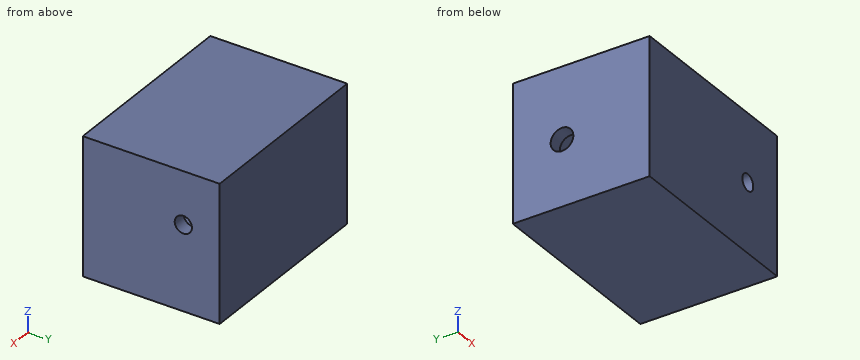
```python
from build123d import *

# Parameters (mm, degrees)
SKETCH1_W           = 70
SKETCH1_H           = 50
BOSS_EXTRUDE1_DEPTH = 50
CUT_EXTRUDE1_START  = -5
SKETCH2_W           = 60
SKETCH2_H           = 40
CUT_EXTRUDE1_DEPTH  = 40
CUT_EXTRUDE2_REACH  = 81.52
SKETCH3_R           = 3
CUT_EXTRUDE3_REACH  = 92.673
SKETCH4_R           = 3.149743794
CUT_EXTRUDE4_REACH  = 92.673
SKETCH5_R           = 4.144549467


with BuildPart() as part:
    # Sketch1 → Boss-Extrude1 (new body)
    with BuildSketch(Plane.XY):
        with Locations((-7.408376963, -3.664921466)):
            Rectangle(SKETCH1_W, SKETCH1_H)
    extrude(amount=BOSS_EXTRUDE1_DEPTH)

    # Sketch2 → Cut-Extrude1 (cut)
    with BuildSketch(Plane(origin=(0, 0, 0), x_dir=(-1, 0, 0), z_dir=(0, 0, -1)).offset(CUT_EXTRUDE1_START)):
        with Locations((7.408376963, -3.664921466)):
            Rectangle(SKETCH2_W, SKETCH2_H)
    extrude(amount=-CUT_EXTRUDE1_DEPTH, mode=Mode.SUBTRACT)

    # Sketch3 → Cut-Extrude2 (cut, up to next)
    with BuildSketch(Plane(origin=(0, -23.664921466, 0), x_dir=(1, 0, 0), z_dir=(0, 1, 0)), mode=Mode.PRIVATE) as cut_extrude2_sk1:
        with Locations(Location((11.436283644, -25.254491461, 0), (0, 0, 270))):
            Circle(SKETCH3_R)
    cut_extrude2_tool1 = extrude(cut_extrude2_sk1.sketch, amount=-CUT_EXTRUDE2_REACH, mode=Mode.PRIVATE) & part.part
    add(cut_extrude2_tool1.solids().sort_by_distance((11.436284, -23.664921, 25.254491))[0], mode=Mode.SUBTRACT)

    # Sketch4 → Cut-Extrude3 (cut, up to next)
    with BuildSketch(Plane(origin=(27.591623037, 0, 0), x_dir=(0, 0, -1), z_dir=(1, 0, 0)), mode=Mode.PRIVATE) as cut_extrude3_sk1:
        with Locations((-30.913262832, 8.056606799)):
            Circle(SKETCH4_R)
    cut_extrude3_tool1 = extrude(cut_extrude3_sk1.sketch, amount=-CUT_EXTRUDE3_REACH, mode=Mode.PRIVATE) & part.part
    add(cut_extrude3_tool1.solids().sort_by_distance((27.591623, 8.056607, 30.913263))[0], mode=Mode.SUBTRACT)

    # Sketch5 → Cut-Extrude4 (cut, up to next)
    with BuildSketch(Plane.ZY.offset(42.408376963), mode=Mode.PRIVATE) as cut_extrude4_sk1:
        with Locations((23.999844242, 3.360492079)):
            Circle(SKETCH5_R)
    cut_extrude4_tool1 = extrude(cut_extrude4_sk1.sketch, amount=-CUT_EXTRUDE4_REACH, mode=Mode.PRIVATE) & part.part
    add(cut_extrude4_tool1.solids().sort_by_distance((-42.408377, 3.360492, 23.999844))[0], mode=Mode.SUBTRACT)


solid = part.part
```
Can you work these out from the model? Positions are in its coordinate system, mm. Give positions to 0.01 mm unless a question says otherwise; leave off trailing zeros. Loops run counter-clockwise (first coordinate to the right, second up) from the corner with the lowest first, then second, coordinate; pieces in that order, holes last. Notation, with made-up numbers: M -6.75,61 L 5.25,61 A7 ccw 5.25,71 Z; hole C 32,71 d9. An arc over 180 degrees is marked long. Answer in a Markdown table with one row per item.
1. Suppose I cut it at B-B on x = -28.5. Write out the boundary of the cut face in (y, z), plus the area to 3 significant figures.
Taken from the geometry:
| item | result |
|---|---|
| outline | M -28.66,0 L 21.34,0 L 21.34,50 L -28.66,50 Z; hole M -23.66,5 L 16.34,5 L 16.34,45 L -23.66,45 Z |
| area | 900 mm² |
2. Suppose I cut it at C-C on z = 33. Write out the boundary of the cut face in (x, y).
Taken from the geometry:
| item | result |
|---|---|
| outline | M -42.41,-28.66 L 27.59,-28.66 L 27.59,5.7 L 22.59,5.7 L 22.59,-23.66 L -37.41,-23.66 L -37.41,16.34 L 22.59,16.34 L 22.59,10.42 L 27.59,10.42 L 27.59,21.34 L -42.41,21.34 Z |
3. If I drill on line 1 along Z through (x, y) = (-30, 12); line 2 along X through (y, z) = (-13, 10); line 3 along Y through (x, z) = (-17, 21), over which ranges is the centre line in solid material (lowest first)?
Taken from the geometry:
| item | result |
|---|---|
| line 1 | z = 0 to 5, 45 to 50 |
| line 2 | x = -42.41 to -37.41, 22.59 to 27.59 |
| line 3 | y = -28.66 to -23.66, 16.34 to 21.34 |
4. Suppose I cut it at A-A on z = 15. Write out the boundary of the cut face in (x, y).
Taken from the geometry:
| item | result |
|---|---|
| outline | M -42.41,-28.66 L 27.59,-28.66 L 27.59,21.34 L -42.41,21.34 Z; hole M -37.41,-23.66 L 22.59,-23.66 L 22.59,16.34 L -37.41,16.34 Z |
